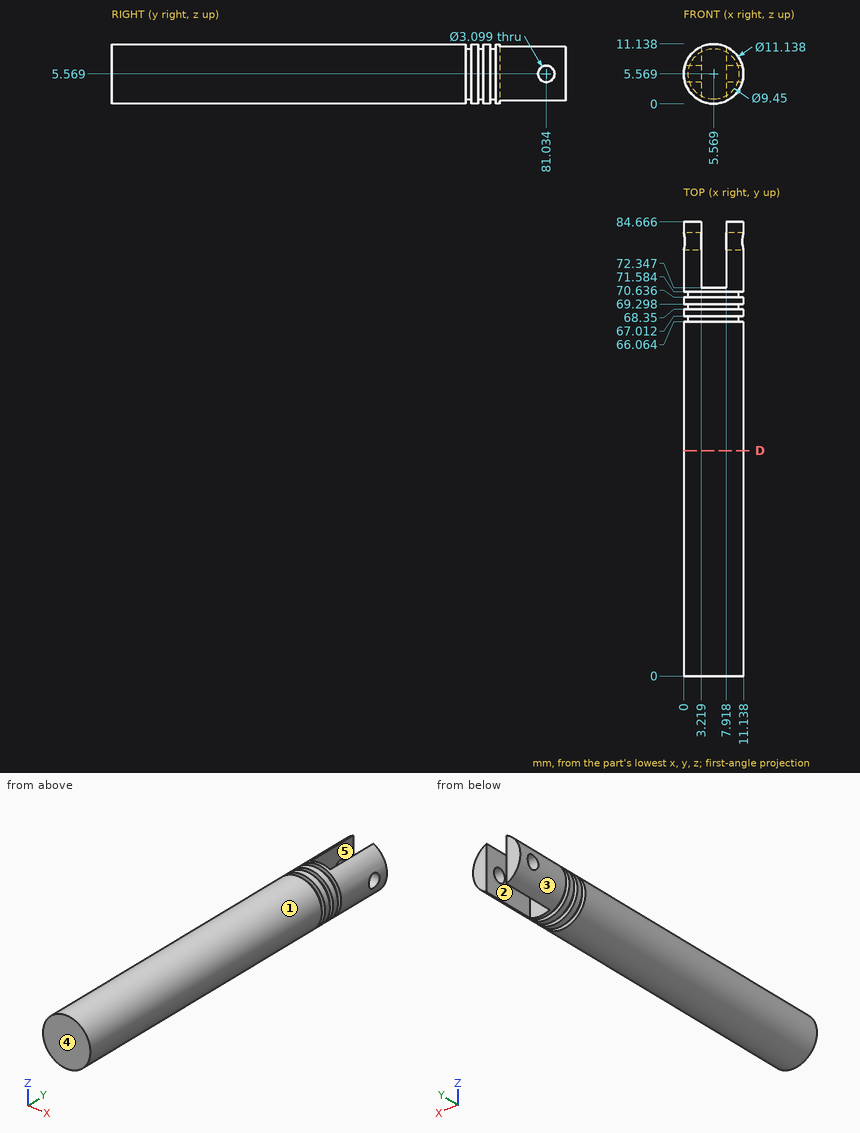
Source: three-view drawing plus pictorial views. Frame: mm from the lowest corner of the part. A direction names the side the tool comes from. Round coordinates to 2 decimals unless told otherwise and drop trailing zeros. Loops run counter-clockwise (first coordinate to the right, second up) from the corner with the lowest first, then second, coordinate; pieces in that order, holes last.
Q1. Access query for the marked faces 1 and 2. Directions: +Z, -Z, +X, -X, +Y, -Y. A direction counts if a zero-diameter tool reaches every point of the face in a straight line with its end or side. Return the directions, or none.
Q2. Section D-D on y = 42. Return loops of the section in (x, z).
Q3. Pull-direction query (X, two-part tool) for the marked faces 3, 4 and 5; classes: released by +X, released by -X, zero draft, split by the parting line, or undercut.
Q4. Pin query (flat end, axial travel): P1, Ø1.5, axis at x = 6.5, z = 10, coming from the +Y side. Return the tip coordinate at first contact, or that it passes through.
Q5. Material intervals for L1, parallel to X at y = 72.5, z = 8.5 (1 decimal); L2, parallel to X at y = 74, z = 7.5 (1 decimal); L3, parallel to Y at x = 7, z = 1.25, sorted ascending.
Evaluation:
1. face 1: +Y, -Y
1. face 2: +Z, -Z, +Y
2. outline: circle Ø11.14 at (5.57, 5.57)
3. face 3: split by the parting line
3. face 4: zero draft
3. face 5: undercut
4. P1: stops at y = 72.35
5. L1: x = 0.8 to 3.2, 7.9 to 10.3
5. L2: x = 0.3 to 3.2, 7.9 to 10.8
5. L3: y = 0 to 72.35
